Part model, mm, in its own coordinate system. Face numbers are marked on the shaded views. A direction names the side the tool comes from. Give positions to 0.01 mm unless a question says otherwise; leave off trailing zeros. Write each loop counter-clockwise with the first axis right and the second up, starting at its lowest first coordinate (ties: lowest second). Pieces come first, ordered by that corner, then holes.
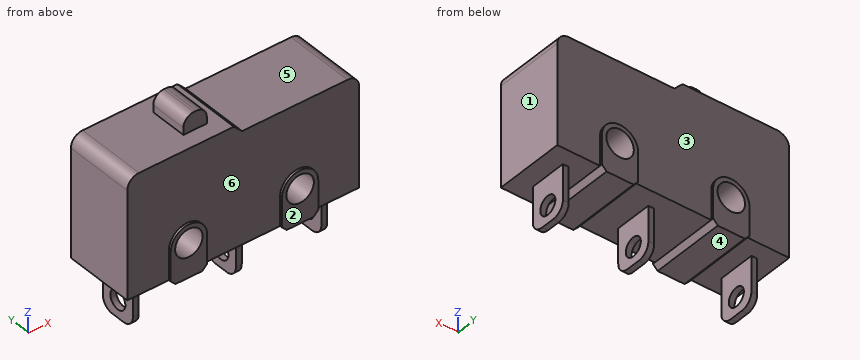
from build123d import *

# Parameters (mm, degrees)
F0_W      = 19.8
F0_H      = 10.2
F1_DEPTH  = 6
F3_DEPTH  = 0.2
F5_DEPTH  = 6.4
F6_DEPTH  = 6.4
F7_SIZE   = 0.39999
F9_DEPTH  = 6.201
F10_R     = 1
F12_D     = 2.35
F14_D     = 2.35
F15_W     = 2
F15_H     = 3.2
F16_DEPTH = 1.5
F17_R     = 0.9
F18_W     = 0.5
F18_H     = 3.2
F19_DEPTH = 4
F21_D     = 1.6
F22_R     = 1


# Not quite as in the source:
# - a fillet or chamfer is up to 0.001 mm smaller than in the source, because OpenCascade refuses the exact size


with BuildPart() as f1:
    # F0 (on Front) → F1 (new body)
    with BuildSketch(Plane.XZ):
        with Locations((9.9, 5.1)):
            Rectangle(F0_W, F0_H)
    extrude(amount=F1_DEPTH)

    # F2 (on face) → F3 (join)
    with BuildSketch(Plane.XZ.offset(6)):
        with BuildLine():
            ThreePointArc((3.55, 2.5), (5.1, 0.95), (6.65, 2.5))
            ThreePointArc((6.65, 2.5), (5.1, 4.05), (3.55, 2.5))
        make_face()
        with BuildLine():
            Line((6.65, -0.4), (6.65, 2.5))
            ThreePointArc((6.65, 2.5), (5.1, 0.95), (3.55, 2.5))
            Line((3.55, 2.5), (3.55, -0.4))
            Line((3.55, -0.4), (6.65, -0.4))
        make_face()
        with BuildLine():
            ThreePointArc((13.05, 2.5), (14.6, 0.95), (16.15, 2.5))
            ThreePointArc((16.15, 2.5), (14.6, 4.05), (13.05, 2.5))
        make_face()
        with BuildLine():
            Line((16.15, -0.4), (16.15, 2.5))
            ThreePointArc((16.15, 2.5), (14.6, 0.95), (13.05, 2.5))
            Line((13.05, 2.5), (13.05, -0.4))
            Line((13.05, -0.4), (16.15, -0.4))
        make_face()
    extrude(amount=F3_DEPTH)

    # F4 (on face) → F5 (join)
    with BuildSketch(Plane.XZ.offset(6.2)):
        with BuildLine():
            Line((6.65, -0.4), (6.65, 2.5))
            ThreePointArc((6.65, 2.5), (5.1, 4.05), (3.55, 2.5))
            Line((3.55, 2.5), (3.55, -0.4))
            Line((3.55, -0.4), (6.65, -0.4))
        make_face()
    extrude(amount=-F5_DEPTH)

    # F6 (add): a face of the model
    f6_faces = [f1.faces().sort_by_distance(p)[0] for p in [
        (14.6, -6.2, 1.6732176073),
    ]]
    extrude(f6_faces, amount=-F6_DEPTH)

    # F7 (size 0.4 in the source; OpenCascade refuses exactly that, so slightly less here)
    f7_edges = [f1.edges().sort_by_distance(p)[0] for p in [
        (3.55, -3, -0.4),
        (6.65, -3, -0.4),
        (13.05, -3, -0.4),
        (16.15, -3, -0.4),
    ]]
    chamfer(f7_edges, length=F7_SIZE)

    # F8 (on face) → F9 (cut, through all)
    with BuildSketch(Plane.XZ.offset(6)):
        Polygon((19.8, 10.2), (9.1, 10.2), (9.8, 9.5), (19.8, 9.5), align=None)
    extrude(amount=-F9_DEPTH, mode=Mode.SUBTRACT)

    # F10
    f10_edges = [f1.edges().sort_by_distance(p)[0] for p in [
        (0, -3, 10.2),
        (19.8, -3, 9.5),
    ]]
    fillet(f10_edges, radius=F10_R)

    # F12 (through all)
    with Locations(Plane.XZ.offset(6.2)):
        with Locations((5.1, 2.5)):
            Hole(F12_D / 2)

    # F14 (through all)
    with Locations(Plane.XZ.offset(6.2)):
        with Locations((14.6, 2.5)):
            Hole(F14_D / 2)

    # F15 (on face) → F16 (join)
    with BuildSketch(Plane.XY.offset(10.2)):
        with Locations((6.9132626522, -3)):
            Rectangle(F15_W, F15_H)
    extrude(amount=F16_DEPTH)

    # F17
    f17_edges = [f1.edges().sort_by_distance(p)[0] for p in [
        (5.913263, -3, 11.7),
        (7.913263, -3, 11.7),
    ]]
    fillet(f17_edges, radius=F17_R)

    # F18 (on face) → F19 (join)
    with BuildSketch(Plane(origin=(0, 0, 0), x_dir=(1, 0, 0), z_dir=(0, 0, -1))):
        with Locations((1.85, 3)):
            Rectangle(F18_W, F18_H)
        with Locations((10.65, 3)):
            Rectangle(F18_W, F18_H)
        with Locations((17.95, 3)):
            Rectangle(F18_W, F18_H)
    extrude(amount=F19_DEPTH)

    # F21 (through all)
    with Locations(Plane(origin=(1.6, 0, 0), x_dir=(0, -1, 0), z_dir=(-1, 0, 0))):
        with Locations((3, -2.4945095647)):
            Hole(F21_D / 2)

    # F22
    f22_edges = [f1.edges().sort_by_distance(p)[0] for p in [
        (17.95, -4.6, -4),
        (10.65, -4.6, -4),
        (1.85, -4.6, -4),
        (1.85, -1.4, -4),
        (10.65, -1.4, -4),
        (17.95, -1.4, -4),
    ]]
    fillet(f22_edges, radius=F22_R)


solid = f1.part
1) Flat gauge pins, fed straight in: P1, Ø1.5, axis at x = 12, y = -1, coming from the +Z side; P2, Ø2.5, axis at x = 4.5, y = -1.5, coming from the -Z side; P3, Ø3, axis at x = 11, z = 2, coming from the +Y side; P4, Ø3, axis at x = 3.5, z = 5, coming from the +Y side. Where does each tip first touch, or does it go through?
Check result:
P1: stops at z = 9.5
P2: stops at z = -0.4
P3: stops at y = 0
P4: stops at y = 0.2
2) Saw through at C-C (x = 5.1). Write the cut outline in (y, z) (3 decimals).
Check result:
outline: (-6.2, -0.4) - (0.2, -0.4) - (0.2, 1.325) - (-6.2, 1.325) - close; (-6.2, 3.675) - (0.2, 3.675) - (0.2, 4.05) - (0, 4.05) - (0, 10.2) - (-6, 10.2) - (-6, 4.05) - (-6.2, 4.05) - close
3) 3-axis set-ups, long thin cutter, end or side, ignore diameter. For the marked faces 4, 5 and 6: which of +Z, -Z, +X, -X, +Y, -Y reach the whole face in a straight line?
Check result:
face 4: -Z, +Y, -Y
face 5: +Z, +X, +Y, -Y
face 6: +Z, -Y
4) Saw through at B-B (x = 14.6). Write the cut outline in (y, z) (3 decimals).
Check result:
outline: (-6.2, -0.4) - (0.2, -0.4) - (0.2, 1.325) - (-6.2, 1.325) - close; (-6.2, 3.675) - (0.2, 3.675) - (0.2, 4.05) - (0, 4.05) - (0, 9.5) - (-6, 9.5) - (-6, 4.05) - (-6.2, 4.05) - close
5) Saw through at D-D (x = 12). Write the cut outline in (y, z).
Check result:
outline: (-6, 0) - (0, 0) - (0, 9.5) - (-6, 9.5) - close
6) Saw through at A-A (y = -5). State how many separate pieces and enclosed holes the cut face has, and give its area (3 significant figures).
Check result:
separate pieces: 1
enclosed holes: 2
area: 188 mm2
7) Drill centre lines: L1, parallel to Z at x = 17.9, y = -3; L2, parallel to Y at x = 6.75, z = 1.5; L3, parallel to Z at x = 5.1, y = -2 (3 decimals). Where is each one in solid material? Low to high.
Check result:
L1: z = -4 to -3.29, -1.69 to 9.5
L2: y = -6 to 0
L3: z = -0.4 to 1.325, 3.675 to 10.2
8) Mould opens along X. For the marked faces 1, 2 and 3 say: +X half, -X half, draft (parallel to the pull), parting line (faces both ways), or undercut.
Check result:
face 1: +X half
face 2: draft
face 3: undercut
